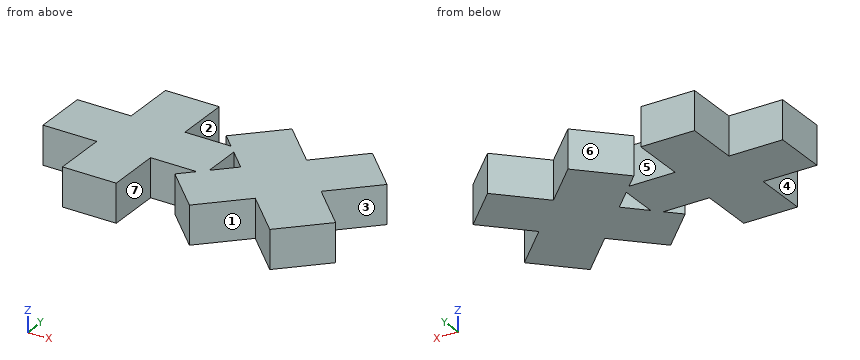
from build123d import *

# Parameters (mm, degrees)
F1_DEPTH = 25


with BuildPart() as f1:
    # F0 (on Top) → F1 (new body)
    with BuildSketch(Plane.XY):
        Polygon((29.8591275221, 42.6615241542), (-5.1408724779, 42.6615241542), (-5.1408724779, 7.6615241542), (-40.1408724779, 7.6615241542), (-40.1408724779, -27.3384758458), (-5.1408724779, -27.3384758458), (-5.1408724779, -62.3384758458), (29.8591275221, -62.3384758458), (29.8591275221, -27.3384758458), (29.8591275221, -9.8384758458), (29.8591275221, 7.6615241542), align=None)
        Polygon((59.8591275221, 7.6615241542), (29.8591275221, 7.6615241542), (29.8591275221, -9.8384758458), (64.8591275221, -9.8384758458), (64.8591275221, 2.6615241542), align=None)
        Polygon((64.8591275221, 7.6615241542), (59.8591275221, 7.6615241542), (64.8591275221, 2.6615241542), align=None)
        Polygon((64.8591275221, -22.3384758458), (59.8591275221, -27.3384758458), (64.8591275221, -27.3384758458), align=None)
        Polygon((64.8591275221, -9.8384758458), (29.8591275221, -9.8384758458), (29.8591275221, -27.3384758458), (59.8591275221, -27.3384758458), (64.8591275221, -22.3384758458), align=None)
        Polygon((51.1961766182, 16.3244750581), (59.8591275221, 7.6615241542), (64.8591275221, 7.6615241542), (64.8591275221, 2.6615241542), (77.3591275221, -9.8384758458), (103.522078426, -9.8384758458), (103.522078426, 16.3244750581), (77.3591275221, 42.4874259621), align=None)
        Polygon((103.522078426, -9.8384758458), (77.3591275221, -9.8384758458), (64.8591275221, -22.3384758458), (64.8591275221, -27.3384758458), (59.8591275221, -27.3384758458), (51.1961766182, -36.0014267497), (77.3591275221, -62.1643776536), (103.522078426, -36.0014267497), align=None)
        Polygon((103.522078426, 16.3244750581), (103.522078426, -9.8384758458), (129.6850293299, -9.8384758458), (155.8479802338, 16.3244750581), (129.6850293299, 42.4874259621), align=None)
        Polygon((129.6850293299, -9.8384758458), (103.522078426, -9.8384758458), (103.522078426, -36.0014267497), (129.6850293299, -62.1643776536), (155.8479802338, -36.0014267497), align=None)
    extrude(amount=F1_DEPTH)


solid = f1.part
Input: part model. Units: mm. Frame: model coordinates. Face numbers are marked on the shaded views. A direction names the side the tool comes from. Round coordinates to 2 decimals unless told otherwise and drop trailing zeros. Write each loop counter-clockwise with the first axis right and the second up, starting at its lowest first coordinate (ties: lowest second). Pieces come first, ordered by that corner, then holes.
1) Contact query for flat-ended pins moving along their axis: P1, Ø7.5, axis at y = -6, z = 16, coming from the +X side; P2, Ø10, axis at y = 1.5, z = 15.5, coming from the +X side; P3, Ø7.5, axis at x = 47, z = 12, coming from the +Y side. Output: stop coordinate, or through.
2) Cut plane C-C (y = -18.5). Return the cut outline in (x, z), then the cut area to 3 significant figures.
3) Cut plane B-B (y = 22). Return the cut outline in (x, z).
4) Cut plane D-D (y = -39.5). Return the cut outline in (x, z).
5) Reachability of the marked faces 4, 5, 6 and 7 from +Z, -Z, +X, -X, +Y, -Y: full face, straight path, thin tool, end or side. Return the list, or none.
6) Draft query along Y for the marked faces 1, 2 and 3. Return one class per face: pulls with the +Y half, pulls with the -Y half, needs draft (parallel to the pull), parting line crosses it, or undercut.
7) Cut plane A-A (z = 15). Return the cut outline in (x, y).
8) Ray query, L1, parallel to X at y = 26.5, z = 11; L2, parallel to X at y = 22.5, z = 5; L3, parallel to Y at x = 56, z = 3. Return the intervals inside material, ascending.
Geometry says:
1. P1: stops at x = 137.27
1. P2: stops at x = 146.02
1. P3: stops at y = 7.66
2. outline: (-40.14, 0) - (64.86, 0) - (64.86, 25) - (-40.14, 25) - close; (68.7, 0) - (138.35, 0) - (138.35, 25) - (68.7, 25) - close
2. area: 4,370 mm2
3. outline: (-5.14, 0) - (29.86, 0) - (29.86, 25) - (-5.14, 25) - close; (56.87, 0) - (97.85, 0) - (97.85, 25) - (56.87, 25) - close; (109.2, 0) - (150.17, 0) - (150.17, 25) - (109.2, 25) - close
4. outline: (-5.14, 0) - (29.86, 0) - (29.86, 25) - (-5.14, 25) - close; (54.69, 0) - (100.02, 0) - (100.02, 25) - (54.69, 25) - close; (107.02, 0) - (152.35, 0) - (152.35, 25) - (107.02, 25) - close
5. face 4: +Z, -Z, -X, -Y
5. face 5: +Z, -Z
5. face 6: +Z, -Z, +Y
5. face 7: +Z, -Z, -Y
6. face 1: pulls with the -Y half
6. face 2: needs draft
6. face 3: undercut
7. outline: (-40.14, -27.34) - (-5.14, -27.34) - (-5.14, -62.34) - (29.86, -62.34) - (29.86, -27.34) - (59.86, -27.34) - (51.2, -36) - (77.36, -62.16) - (103.52, -36) - (129.69, -62.16) - (155.85, -36) - (129.69, -9.84) - (155.85, 16.32) - (129.69, 42.49) - (103.52, 16.32) - (77.36, 42.49) - (51.2, 16.32) - (59.86, 7.66) - (29.86, 7.66) - (29.86, 42.66) - (-5.14, 42.66) - (-5.14, 7.66) - (-40.14, 7.66) - close; hole (64.86, -22.34) - (77.36, -9.84) - (64.86, 2.66) - close
8. L1: x = -5.14 to 29.86, 61.37 to 93.35, 113.7 to 145.67
8. L2: x = -5.14 to 29.86, 57.37 to 97.35, 109.7 to 149.67
8. L3: y = -40.81 to -31.2, -27.34 to 7.66, 11.52 to 21.13
